Verification items for the finished model (mm, model axes). A direction names the side the tool comes from. Give positions to 0.01 mm unless a question says otherwise; leave off trailing zeros. Loops run counter-clockwise (first coordinate to the right, second up) from the corner with the lowest first, then second, coordinate; pieces in that order, holes last. Notation, with made-up numbers: M 42.25,-6.5 L 65.25,-6.5 A35 ccw 65.25,31.5 Z; hole C 8.25,68 d8. An arc over 180 degrees is marked long. Use a Markdown table: item, result.
from build123d import *

# Parameters (mm, degrees)
DODANIE_WYCI_GNI_CIE1_DEPTH = 6
SZKIC2_W                    = 3.003669228
SZKIC2_H                    = 1.997379701
DODANIE_WYCI_GNI_CIE2_DEPTH = 2
SZKIC3_W                    = 3.00029081
SZKIC3_H                    = 1.99738112
DODANIE_WYCI_GNI_CIE3_DEPTH = 2


with BuildPart() as part:
    # Szkic1 → Dodanie-wyciągnięcie1 (new body)
    with BuildSketch(Plane.XY):
        Polygon((0, -199.086972688), (0, -197.089592987), (-8, -197.089592987), (-7.997619842, -199.086972688), align=None)
    extrude(amount=-DODANIE_WYCI_GNI_CIE1_DEPTH)

    # Szkic2 → Dodanie-wyciągnięcie2 (add)
    with BuildSketch(Plane(origin=(0, 0, 0), x_dir=(0, 0, -1), z_dir=(1, 0, 0))):
        with Locations((3.49731299, -198.088282838)):
            Rectangle(SZKIC2_W, SZKIC2_H)
    extrude(amount=DODANIE_WYCI_GNI_CIE2_DEPTH)

    # Szkic3 → Dodanie-wyciągnięcie3 (add)
    with BuildSketch(Plane(origin=(-8.234848226, -0.009812978, 0), x_dir=(0, 0, 1), z_dir=(-0.99999929, -0.00119164, 0))):
        with Locations((-3.499897311, -198.078610496)):
            Rectangle(SZKIC3_W, SZKIC3_H)
    extrude(amount=DODANIE_WYCI_GNI_CIE3_DEPTH)


solid = part.part
(1) Material ranges on line 1 (X direction, y = -197.95, z = -1.9); line 2 (Y direction, x = -3, z = -2.95); line 3 (X direction, y = -198.55, z = -3.75), recorded low to high.
Results below:
| item | result |
|---|---|
| line 1 | -8 to 0 |
| line 2 | -199.09 to -197.09 |
| line 3 | -10 to 2 |
(2) Cross-section at A-A on y = -197.4. Record the cut outline in (x, z), then the cut area to 3 significant figures.
Results below:
| item | result |
|---|---|
| outline | M -10,-5 L -8,-5 L -8,-6 L 0,-6 L 0,-5 L 2,-5 L 2,-2 L 0,-2 L 0,0 L -8,0 L -8,-2 L -10,-2 Z |
| area | 60.0 mm^2 |
(3) Set-up check for faces 1 (the flat face through (-9, -198, -2)), 2 (the flat face through (-4, -198, 0)), 3 (the flat face through (-9, -198, -5)), 4 (the flat face through (1, -198, -4.999)), 5 (the flat face through (1, -198, -1.995)): record each of +Z, -Z, +X, -X, +Y, -Y from which the full face is reachable in a straight line by a thin tool's end or side.
Results below:
| item | result |
|---|---|
| face 1 | +Z, -X, +Y, -Y |
| face 2 | +Z, +X, -X, +Y, -Y |
| face 3 | -Z, -X, +Y, -Y |
| face 4 | -Z, +X, +Y, -Y |
| face 5 | +Z, +X, +Y, -Y |
(4) Cross-section at B-B on z = -1.75. Record the cut outline in (x, y).
Results below:
| item | result |
|---|---|
| outline | M -8,-199.09 L 0,-199.09 L 0,-197.09 L -8,-197.09 Z |
(5) Gauge pin test, flat ends, axial feed: P1, Ø1, axis at x = 1.5, y = -198, coming from the +Z side; P2, Ø0.8, axis at y = -198, z = -5.5, coming from the +X side. Record the tip position at first contact, or that the pin passes through.
Results below:
| item | result |
|---|---|
| P1 | z = -2 |
| P2 | x = 0 |
